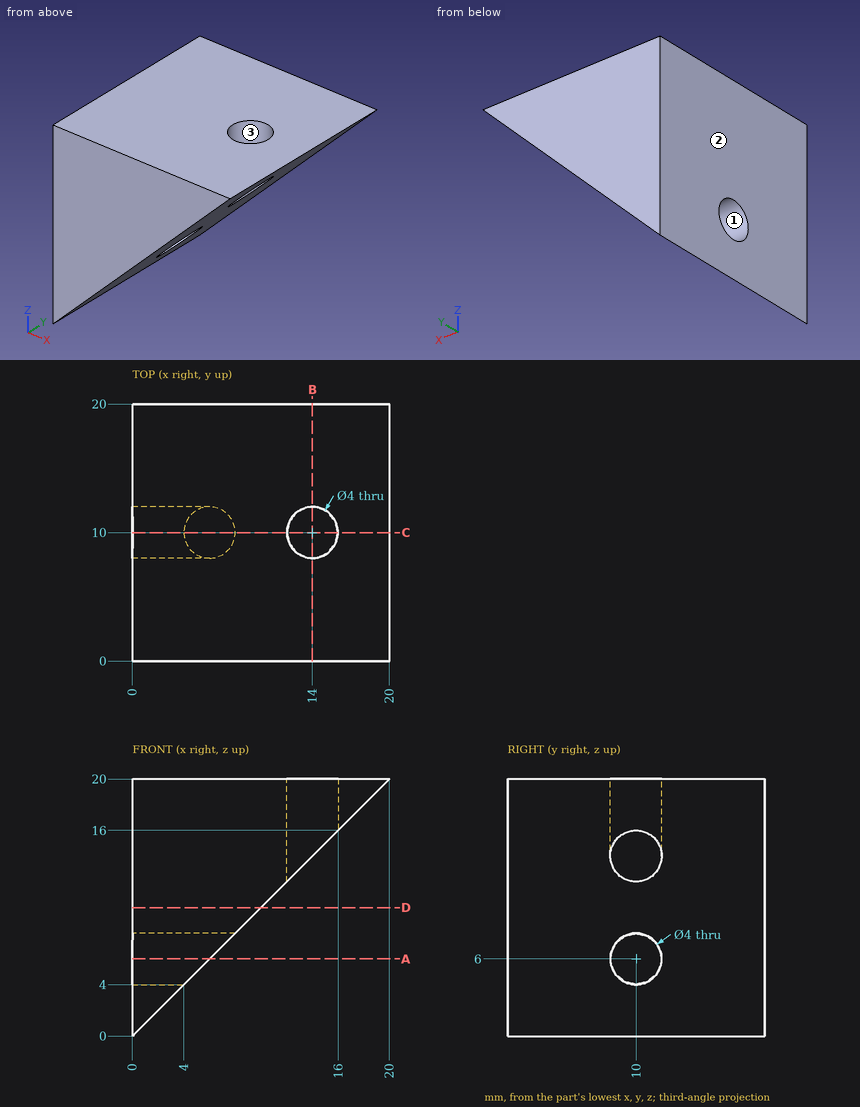
Part print with two shaded views. Sizes in mm from the minimum x, y, z corner. Coordinates: 2 decimals unless noted, no trailing zeros. Write each loop counter-clockwise with the first axis right and the second up, starting at its lowest first coordinate (ties: lowest second). Pieces come first, ordered by that corner, then holes. Notation, with made-up numbers: (17, -19.75) - (62, -19.75) arc R22 cw to (62, 6.25) - close; hole circle Ø1 at (33, 67). An arc over 180 degrees is marked (long way). One line per item, written item: value. Start each with the question number.
1. Slice it at B-B (x = 14). Write the cut outline in (y, z), plus the area to 3 significant figures.
2. Slice it at D-D (z = 10). Write the cut outline in (x, y), plus the area to 3 significant figures.
3. Flat gauge pins, fed straight in: pin 1 (3 mm diameter, centred on x = 14, y = 10, fed in from +Z); pin 2 (1.5 mm diameter, centred on y = 8, z = 17, fed in from +X); pin 3 (1.5 mm diameter, centred on y = 16.5, z = 5.5, fed in from +X). Where does each tip first touch, or does it go through?
4. Slice it at A-A (z = 6). Write the cut outline in (x, y).
5. Slice it at C-C (y = 10). Write the cut outline in (x, z), plus the area to 3 significant figures.
6. Probe line 1 (Y direction, x = 14, z = 17.75); line 2 (X direction, y = 10, z = 15.5); line 3 (Z direction, x = 6.75, y = 10). List the from-to ranges inside material, lowest first. Write a range as from..to.
7. Mould opens along X. For the marked faces 1, 2 and 3 say: released by +X, released by -X, zero draft, split by the parting line, or undercut.
Answers below:
1. outline: (0, 14) - (8, 14) - (8, 20) - (0, 20) - close; (12, 14) - (20, 14) - (20, 20) - (12, 20) - close
1. area: 96.0 mm^2
2. outline: (0, 0) - (10, 0) - (10, 20) - (0, 20) - close
2. area: 200 mm^2
3. pin 1: passes through
3. pin 2: stops at x = 17.75
3. pin 3: stops at x = 6.25
4. outline: (0, 0) - (6, 0) - (6, 8) - (0, 8) - close; (0, 12) - (6, 12) - (6, 20) - (0, 20) - close
5. outline: (0, 0) - (4, 4) - (0, 4) - close; (0, 8) - (8, 8) - (12, 12) - (12, 20) - (0, 20) - close; (16, 16) - (20, 20) - (16, 20) - close
5. area: 152 mm^2
6. line 1: y = 0..8, 12..20
6. line 2: x = 0..12
6. line 3: z = 8..20
7. face 1: zero draft
7. face 2: released by -X
7. face 3: undercut
